from build123d import *

# Parameters (mm, degrees)
SKETCH1_W                = 533.4
SKETCH1_H                = 38.1
BOSS_EXTRUDE1_DEPTH      = 6.35
SKETCH2_R                = 11
CUT_EXTRUDE1_DEPTH       = 7.62
F_0_257_DIAMETER_HOLE1_D = 6.5278


with BuildPart() as part:
    # Sketch1 → Boss-Extrude1 (new body)
    with BuildSketch(Plane(origin=(0, 0, 0), x_dir=(1, 0, 0), z_dir=(0, 1, 0))):
        Rectangle(SKETCH1_W, SKETCH1_H)
    extrude(amount=BOSS_EXTRUDE1_DEPTH)

    # Sketch2 → Cut-Extrude1 (cut)
    with BuildSketch(Plane(origin=(0, 6.35, 0), x_dir=(1, 0, 0), z_dir=(0, 1, 0))):
        Circle(SKETCH2_R)
    extrude(amount=-CUT_EXTRUDE1_DEPTH, mode=Mode.SUBTRACT)

    # F (0.257) Diameter Hole1 (through all)
    with Locations(Plane(origin=(0, 6.35, 0), x_dir=(1, 0, 0), z_dir=(0, 1, 0))):
        with Locations((234.95, 0), (196.85, 0)):
            f_0_257_diameter_hole1 = Hole(F_0_257_DIAMETER_HOLE1_D / 2)

    # Mirror1: F (0.257) Diameter Hole1 across plane
    add(f_0_257_diameter_hole1.mirror(Plane(origin=(0, 0, 0), x_dir=(0, 0, 1), z_dir=(1, 0, 0))), mode=Mode.SUBTRACT)


solid = part.part
The model under review builds one solid part; all positions refer to its coordinate system, in mm. Give positions to 0.01 mm unless a question says otherwise; leave off trailing zeros. Loops run counter-clockwise (first coordinate to the right, second up) from the corner with the lowest first, then second, coordinate; pieces in that order, holes last. Notation, with made-up numbers: (86, 43) -> (95, 43) arc R14 cw to (95, 53) -> close; hole circle Ø8 at (-12.75, -18.75). An arc over 180 degrees is marked (long way). Answer as a JSON object with one key per item and string values. Group by question number.
Q1. Draft analysis for pull direction X (two halves, no side actions). For faces 1 (the flat face through (-4, 6.35, 12)), 2 (the cylindrical face through (-2.38, 3.22, 10.74)), state which applies: pulls with the +X half, pulls with the -X half, needs draft (parallel to the pull), parting line crosses it, or undercut.
Q2. Wall thickness on line 1 along Z through (x, y) = (-196.85, 2.5); line 2 along Z through (x, y) = (0, 2.25); line 3 along X through (y, z) = (6, 2): over which ranges is each line inside the solid? List them lowest first.
Q3. Take a section at B-B (y = 1.5). Write out the cut boundary in (x, z).
Q4. Take a section at A-A (x = 0). Write out the cut boundary in (y, z).
Q5. Insertion check: pin 1 (10.5 mm diameter, centred on x = 196.85, z = 0, fed in from -Y). The pin has a flat end and moves straight along its axis. Give the tip position at first contact, or say it passes through.
Answer below:
{
 "1": {"face 1": "needs draft", "face 2": "undercut"},
 "2": {"line 1": "z = -19.05 to -3.26, 3.26 to 19.05", "line 2": "z = -19.05 to -11, 11 to 19.05", "line 3": "x = -266.7 to -237.53, -232.37 to -199.43, -194.27 to -10.82, 10.82 to 194.27, 199.43 to 232.37, 237.53 to 266.7"},
 "3": {"outline": "(-266.7, -19.05) -> (266.7, -19.05) -> (266.7, 19.05) -> (-266.7, 19.05) -> close; hole circle Ø6.53 at (-234.95, 0); hole circle Ø6.53 at (-196.85, 0); hole circle Ø22 at (0, 0); hole circle Ø6.53 at (196.85, 0); hole circle Ø6.53 at (234.95, 0)"},
 "4": {"outline": "(0, -19.05) -> (6.35, -19.05) -> (6.35, -11) -> (0, -11) -> close; (0, 11) -> (6.35, 11) -> (6.35, 19.05) -> (0, 19.05) -> close"},
 "5": {"pin 1": "stops at y = 0"}
}
